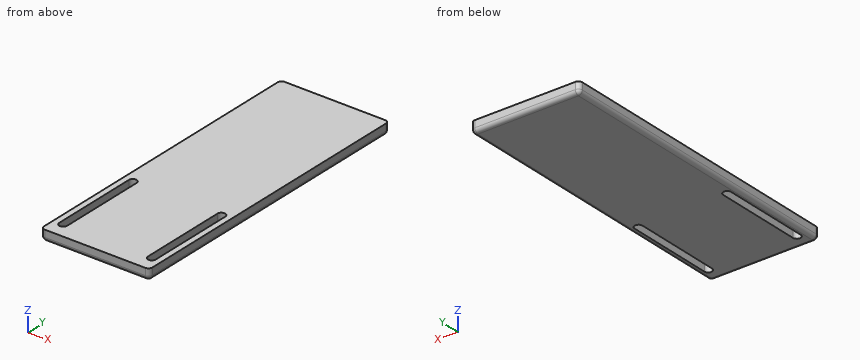
Autodesk Inventor part; units mm, degrees
ref_plane "YZ Plane" through (0, 0, 0) normal (1, 0, 0) x (0, 1, 0)
ref_plane "XZ Plane" through (0, 0, 0) normal (0, 1, 0) x (-1, 0, 0)
ref_plane "XY Plane" through (0, 0, 0) normal (0, 0, 1) x (1, 0, 0)
sketch "Sketch1" plane through (0, 0, 0) normal (0, 0, 1) x (1, 0, 0)
  line L0 (4.8895, 31.75) -> (-4.8895, 31.75)
  line L1 (-4.8895, 31.75) -> (-4.8895, -31.75)
  line L2 (-4.8895, -31.75) -> (4.8895, -31.75)
  line L3 (4.8895, -31.75) -> (4.8895, 31.75)
  line L4 (-4.8895, -31.75) -> (-59.8895, -31.75)
  line L5 (-59.8895, -31.75) -> (-59.8895, 93.25)
  line L6 (-59.8895, 93.25) -> (-4.8895, 93.25)
  line L7 (-4.8895, 93.25) -> (-4.8895, -31.75)
  point P0 (0, 0)
  dimension "d0" = 125
  dimension "d1" = 55
extrude "Extrusion1" add sketch "Sketch1" against normal blind 5.5 contours L1 L4 L5 L6 L7
sketch "Sketch3" plane through (-59.8895, -31.75, 0) normal (0, -1, 0) x (1, 0, 0)
  line L0 (0, 0) -> (55, 0)
  line L1 (0, 0) -> (0, -5.5)
  line L2 (55, -5.5) -> (0, -5.5)
  line L3 (55, 0) -> (55, -5.5)
  point P0 (59.8895, 0)
extrude "Extrusion2" add sketch "Sketch3" along normal blind 30
sketch "Sketch4" plane through (0, 0, -5.5) normal (0, 0, -1) x (-1, 0, 0)
  circle A0 centre (54.8895, -8.75) radius 1.25
  circle A1 centre (9.8895, -8.75) radius 1.25
  circle A2 centre (54.8895, -8.75) radius 2
  circle A3 centre (9.8895, -8.75) radius 2
  line L0 (9.8895, -8.75) -> (9.8895, -53.75)
  circle A4 centre (9.8895, -53.75) radius 2
  line L1 (54.8895, -8.75) -> (54.8895, -53.75)
  circle A5 centre (54.8895, -53.75) radius 2
  line L2 (56.8895, -8.75) -> (52.8895, -8.75)
  line L3 (52.8895, -8.75) -> (52.8895, -53.75)
  line L4 (52.8895, -53.75) -> (56.8895, -53.75)
  line L5 (56.8895, -53.75) -> (56.8895, -8.75)
  line L6 (11.8895, -8.75) -> (7.8895, -8.75)
  line L7 (7.8895, -8.75) -> (7.8895, -53.75)
  line L8 (7.8895, -53.75) -> (11.8895, -53.75)
  line L9 (11.8895, -53.75) -> (11.8895, -8.75)
  point P0 (0, 0)
  dimension "d6" = 4
  dimension "d7" = 4
  dimension "d9" = 4
  dimension "d11" = 4
  dimension "d8" = 45
  dimension "d10" = 45
extrude "Extrusion3" cut sketch "Sketch4" against normal blind 30
fillet "Fillet1" radius 2 4 edges at (-59.8895, 93.25, -2.75) (-4.8895, 93.25, -2.75) (-4.8895, -61.75, -2.75) (-59.8895, -61.75, -2.75)
fillet "Fillet2" radius 2 6 edges at (-4.8895, 15.75, -5.5) (-5.4753, 92.6642, -5.5) (-32.3895, 93.25, -5.5) (-59.3037, 92.6642, -5.5) (-59.8895, 15.75, -5.5) (-32.3895, -61.75, -5.5)
properties part number "HeadBase"
The model under review builds one solid part; all positions refer to its coordinate system, in mm. Give positions to 0.01 mm unless a question says otherwise; leave off trailing zeros. Write each loop counter-clockwise with the first axis right and the second up, starting at its lowest first coordinate (ties: lowest second). Pieces come first, ordered by that corner, then holes.
(1) To check wall thickness, follow L1, parallel to X at y = -17, z = -3.4; L2, parallel to Y at x = -47, z = -3.6; L3, parallel to X at y = 47, z = -3.8. State the ranges of each line that lie inside material, in increasing order.
(2) Consider section A-A, the plane y = -40.5. Give the boundary of the cut face in (x, z), and give its area (3 significant figures).
(3) For P1, Ø2, axis at y = 62, z = -5, coming from the -X side, flat-tipped, find the tip position at first contact; note if it passes through.
(4) Consider section B-B, the plane z = -1.4. Give the boundary of the cut face in (x, y), and give its area (3 significant figures).
Returned:
1. L1: x = -59.89 to -56.89, -52.89 to -11.89, -7.89 to -4.89
1. L2: y = -61.75 to 93.25
1. L3: x = -59.87 to -4.91
2. outline: (-59.89, -3.5) arc R2 ccw to (-57.89, -5.5) - (-56.89, -5.5) - (-56.89, 0) - (-59.89, 0) - close; (-52.89, -5.5) - (-11.89, -5.5) - (-11.89, 0) - (-52.89, 0) - close; (-7.89, -5.5) - (-6.89, -5.5) arc R2 ccw to (-4.89, -3.5) - (-4.89, 0) - (-7.89, 0) - close
2. area: 257 mm2
3. P1: stops at x = -59.83
4. outline: (-59.89, -59.75) arc R2 ccw to (-57.89, -61.75) - (-6.89, -61.75) arc R2 ccw to (-4.89, -59.75) - (-4.89, 91.25) arc R2 ccw to (-6.89, 93.25) - (-57.89, 93.25) arc R2 ccw to (-59.89, 91.25) - close; hole (-56.89, -53.75) arc R2 ccw to (-52.89, -53.75) - (-52.89, -8.75) arc R2 ccw to (-56.89, -8.75) - close; hole (-11.89, -53.75) arc R2 ccw to (-7.89, -53.75) - (-7.89, -8.75) arc R2 ccw to (-11.89, -8.75) - close
4. area: 8,140 mm2
